```python
from build123d import *

# Parameters (mm, degrees)
F1_DEPTH = 228.6
F2_R     = 5
F3_DEPTH = 25
F4_R     = 5
F5_DEPTH = 101.601


with BuildPart() as f1:
    # F0 (on Front) → F1 (new body)
    with BuildSketch(Plane.XZ):
        Polygon((-84.627599, 51.257959), (-97.327599, 51.257959), (-97.327599, -113.342041), (4.272401, -113.342041), (4.272401, -100.642041), (-84.627599, -100.642041), align=None)
    extrude(amount=F1_DEPTH)

    # F2 (on face) → F3 (cut)
    with BuildSketch(Plane(origin=(0, 0, -113.342041), x_dir=(1, 0, 0), z_dir=(0, 0, -1))):
        with Locations((-3.013599, 172.19039)):
            Circle(F2_R)
        with Locations((-3.013599, 56.40959)):
            Circle(F2_R)
        with Locations((-75.014999, 172.19039)):
            Circle(F2_R)
        with Locations((-75.014999, 56.40959)):
            Circle(F2_R)
        with Locations((-75.014999, 15.875)):
            Circle(F2_R)
        with Locations((-75.014999, 212.725)):
            Circle(F2_R)
    extrude(amount=-F3_DEPTH, mode=Mode.SUBTRACT)

    # F4 (on face) → F5 (cut, through all)
    with BuildSketch(Plane(origin=(-97.327599, 0, 0), x_dir=(0, -1, 0), z_dir=(-1, 0, 0))):
        with Locations((200.8924, 8.057959)):
            Circle(F4_R)
        with Locations((128.8924, 8.057959)):
            Circle(F4_R)
        with Locations((99.7076, 8.057959)):
            Circle(F4_R)
        with Locations((27.7076, 8.057959)):
            Circle(F4_R)
        with Locations((27.708, -64.942041)):
            Circle(F4_R)
        with Locations((99.708, -64.942041)):
            Circle(F4_R)
        with Locations((128.892, -64.942041)):
            Circle(F4_R)
        with Locations((200.892, -64.942041)):
            Circle(F4_R)
    extrude(amount=-F5_DEPTH, mode=Mode.SUBTRACT)


solid = f1.part
```
The model under review builds one solid part; all positions refer to its coordinate system, in mm. A direction names the side the tool comes from. Round coordinates to 2 decimals unless told otherwise and drop trailing zeros. Write each loop counter-clockwise with the first axis right and the second up, starting at its lowest first coordinate (ties: lowest second). Pieces come first, ordered by that corner, then holes. Notation, with made-up numbers: (18.25, 11.5) - (38.25, 11.5) arc R12 ccw to (38.25, 23.5) - close; hole circle Ø5 at (-27.5, 66.25). An arc over 180 degrees is marked (long way). Use one line per item in the form item = value.
Q1. Consider section A-A (x = -77). State the section outline as (y, z) points.
Answer key:
outline = (-228.6, -113.34) - (-217.31, -113.34) - (-217.31, -100.64) - (-228.6, -100.64) - close; (-208.14, -113.34) - (-176.78, -113.34) - (-176.78, -100.64) - (-208.14, -100.64) - close; (-167.6, -113.34) - (-61, -113.34) - (-61, -100.64) - (-167.6, -100.64) - close; (-51.82, -113.34) - (-20.46, -113.34) - (-20.46, -100.64) - (-51.82, -100.64) - close; (-11.29, -113.34) - (0, -113.34) - (0, -100.64) - (-11.29, -100.64) - close
Q2. For line 1 (Z direction, x = -34.5, y = -190); line 2 (X direction, y = -65, z = -66), list the stretches that pass through material, from the lowest coordinate up. Write a range as [from, to].
Answer key:
line_1 = [-113.34, -100.64]
line_2 = [-97.33, -84.63]
Q3. Insertion check: pin 1 Ø8 at (y, z) = (-27.71, -64.94) entering from -X; pin 2 Ø16 at (y, z) = (-99.71, -64.94) entering from +X; pin 3 Ø11.5 at (x, y) = (-75.01, -172.19) entering from +Z. Each pin has a flat end and moves straight along its axis. Give the tip position at first contact, or say it passes through.
Answer key:
pin_1 = through
pin_2 = -84.63
pin_3 = -100.64
Q4. Draft analysis for pull direction Z (two halves, no side actions). For faces 1 (the flat face through (-91, -113, 51.258)), 2 (the cylindrical face through (-91.066, -195.897, -64.722)), 3 (the flat face through (-88, 0, -55)), state which applies: +Z half, -Z half, draft (parallel to the pull), parting line (faces both ways), or undercut.
Answer key:
face_1 = +Z half
face_2 = undercut
face_3 = draft
Q5. Consider section B-B (y = -102). State the section outline as (x, z) points.
Answer key:
outline = (-97.33, -113.34) - (4.27, -113.34) - (4.27, -100.64) - (-84.63, -100.64) - (-84.63, -69.39) - (-97.33, -69.39) - close; (-97.33, -60.5) - (-84.63, -60.5) - (-84.63, 3.61) - (-97.33, 3.61) - close; (-97.33, 12.5) - (-84.63, 12.5) - (-84.63, 51.26) - (-97.33, 51.26) - close
Q6. Consider section C-C (z = -77.5). State the section outline as (x, y) points, and give its area (3 significant figures).
Answer key:
outline = (-97.33, -228.6) - (-84.63, -228.6) - (-84.63, 0) - (-97.33, 0) - close
area = 2,900 mm2
Q7. Consider section D-D (y = -36). State the section outline as (x, z) points.
Answer key:
outline = (-97.33, -113.34) - (4.27, -113.34) - (4.27, -100.64) - (-84.63, -100.64) - (-84.63, 51.26) - (-97.33, 51.26) - close
Q8. Tool access review of faces 4 (the flat face through (-84.628, -113, -26)), 5 (the flat face through (-47, -113, -113.342)): name each direction out of +Z, -Z, +X, -X, +Y, -Y from which nothing blocks a thin tool from reaching the whole face with its end or side.
Answer key:
face_4 = +Z, +X, +Y, -Y
face_5 = -Z, +X, -X, +Y, -Y
